```python
from build123d import *

# Parameters (mm, degrees)
F1_DEPTH = 6.35
F2_W     = 3.81
F2_H     = 69.85
F3_DEPTH = 5.08
F5_DEPTH = 25.4


with BuildPart() as f1:
    # F0 (on Front) → F1 (new body)
    with BuildSketch(Plane.XZ):
        with BuildLine():
            ThreePointArc((38.1, 72.39), (36.984077, 75.084077), (34.29, 76.2))
            Line((34.29, 76.2), (-34.29, 76.2))
            ThreePointArc((-34.29, 76.2), (-36.984077, 75.084077), (-38.1, 72.39))
            Line((-38.1, 72.39), (-38.1, -72.39))
            ThreePointArc((-38.1, -72.39), (-36.984077, -75.084077), (-34.29, -76.2))
            Line((-34.29, -76.2), (34.29, -76.2))
            ThreePointArc((34.29, -76.2), (36.984077, -75.084077), (38.1, -72.39))
            Line((38.1, -72.39), (38.1, 72.39))
        make_face()
    extrude(amount=F1_DEPTH)

    # F2 (on face) → F3 (join)
    with BuildSketch(Plane.XZ.offset(6.35)):
        with Locations((32.262094, 0)):
            Rectangle(F2_W, F2_H)
    extrude(amount=F3_DEPTH)

    # F4 (on face) → F5 (cut)
    with BuildSketch(Plane(origin=(30.357094, 0, 0), x_dir=(0, -1, 0), z_dir=(-1, 0, 0))):
        Polygon((6.35, 27.559), (6.35, 0), (6.35, -27.559), (8.89, -27.559), (8.89, 27.559), align=None)
    extrude(amount=-F5_DEPTH, mode=Mode.SUBTRACT)


solid = f1.part
```
CAD build for the part. Positions are in the model's coordinates, mm. A direction names the side the tool comes from. Coordinates: 2 decimals unless noted, no trailing zeros. Loops run counter-clockwise (first coordinate to the right, second up) from the corner with the lowest first, then second, coordinate; pieces in that order, holes last. Notation, with made-up numbers: (10, 13) - (28, 13) arc R19 ccw to (28, 43) - close; hole circle Ø4 at (60, 88). An arc over 180 degrees is marked (long way). Use CSV: the item, a comma, the result in double quotes. Start each with the question number.
Q1. Cut at B-B, the plane x = -28.5. List the corners of the cut face in (y, z), then the cut area to 3 significant figures.
Q2. Cut at A-A, the plane z = 15.5. List the corners of the cut face in (x, y).
Q3. Two-plate mould, pull along Y, no slides. Class faces 6 (the flat face through (-1, 0, 1)), 7 (the flat face through (32, -8.89, 0)), 8 (the flat face through (32, -9, -34.925)): +Y half, -Y half, draft (parallel to the pull), parting line (faces both ways), or undercut.
Q4. 3-axis set-ups, long thin cutter, end or side, ignore diameter. For faces 1 (the flat face through (34.167, -10, 0)), 2 (the flat face through (0, -3, -76.2)), 3 (the flat face through (30.357, -10, 0)), 4 (the flat face through (32, -9, 34.925)), 5 (the flat face through (38.1, -3, -1)): which of +Z, -Z, +X, -X, +Y, -Y reach the whole face in a straight line?
Q5. Cut at C-C, the plane z = -62. List the corners of the cut face in (x, y).
Q6. Drop flat-ended pins along their axis: P1, Ø0.8, axis at x = 32, y = -7.5, coming from the +Z side (3 decimals); P2, Ø3, axis at x = 32, y = -9.5, coming from the -Z side (3 decimals); P3, Ø23, axis at x = 18, z = -11, coming from the -Y side; P4, Ø5, axis at y = -10, z = 38.5, coming from the -X side. Give the stop position or say it passes through.
Q7. Probe probe 1 along Z at (x, y) = (31, -8.75) (3 decimals); probe 2 along Y at (x, z) = (-14.5, -60.5); probe 3 along X at (y, z) = (-10.25, 19.5). List the from-to ranges inside material, lowest first. Write a range as from..to.
Here are the results:
1,outline,"(-6.35, -76.2) - (0, -76.2) - (0, 76.2) - (-6.35, 76.2) - close"
1,area,"968 mm2"
2,outline,"(-38.1, -6.35) - (38.1, -6.35) - (38.1, 0) - (-38.1, 0) - close; (30.36, -11.43) - (34.17, -11.43) - (34.17, -8.89) - (30.36, -8.89) - close"
3,face 6,"+Y half"
3,face 7,"undercut"
3,face 8,"draft"
4,face 1,"+Z, -Z, +X, -Y"
4,face 2,"-Z, +X, -X, +Y, -Y"
4,face 3,"+Z, -Z, -X, -Y"
4,face 4,"+Z, +X, -X, -Y"
4,face 5,"+Z, -Z, +X, +Y, -Y"
5,outline,"(-38.1, -6.35) - (38.1, -6.35) - (38.1, 0) - (-38.1, 0) - close"
6,P1,"z = 34.925"
6,P2,"z = -34.925"
6,P3,"y = -6.35"
6,P4,"through"
7,probe 1,"-34.925..-27.559, 27.559..34.925"
7,probe 2,"-6.35..0"
7,probe 3,"30.36..34.17"
